Verification items for the finished model (mm, model axes). Face numbers are marked on the shaded views. A direction names the side the tool comes from. Coordinates: 2 decimals unless noted, no trailing zeros. Order: outer loops, then holes, each group sorted by start corner. A loop starts at its lowest first (then second) coordinate and runs counter-clockwise, first axis right, second up. Notation, with made-up numbers: (85.25, 48) -> (137.25, 48) arc R17 ccw to (137.25, 75) -> close; hole circle Ø9 at (-14, 66). An arc over 180 degrees is marked (long way). Answer as CSV lines item,"result".
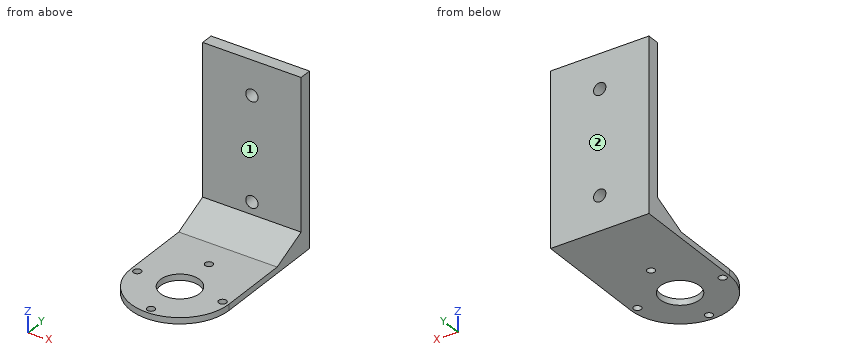
```python
from build123d import *

# Parameters (mm, degrees)
SKETCH1_R           = 10.16
SKETCH1_R_2         = 2
BOSS_EXTRUDE1_DEPTH = 3.175
SKETCH2_W           = 50.8
SKETCH2_H           = 88.9
SKETCH2_R           = 3.175
BOSS_EXTRUDE2_DEPTH = 6.35
BOSS_EXTRUDE3_DEPTH = 50.8


with BuildPart() as part:
    # Sketch1 → Boss-Extrude1 (new body)
    with BuildSketch(Plane.XY):
        with BuildLine():
            Line((-25.4, 0), (-25.4, 60.96))
            Line((-25.4, 60.96), (25.4, 60.96))
            Line((25.4, 60.96), (25.4, 0))
            ThreePointArc((25.4, 0), (0, -25.4), (-25.4, 0))
        make_face()
        Circle(SKETCH1_R, mode=Mode.SUBTRACT)
        with Locations((0, -22)):
            Circle(SKETCH1_R_2, mode=Mode.SUBTRACT)
        with Locations((-22, 0)):
            Circle(SKETCH1_R_2, mode=Mode.SUBTRACT)
        with Locations((0, 22)):
            Circle(SKETCH1_R_2, mode=Mode.SUBTRACT)
        with Locations((22, 0)):
            Circle(SKETCH1_R_2, mode=Mode.SUBTRACT)
    extrude(amount=BOSS_EXTRUDE1_DEPTH)

    # Sketch2 → Boss-Extrude2 (add)
    with BuildSketch(Plane(origin=(0, 60.96, 0), x_dir=(1, 0, 0), z_dir=(0, 1, 0))):
        with Locations((0, -44.45)):
            Rectangle(SKETCH2_W, SKETCH2_H)
        with Locations(Location((0, -17.78, 0), (0, 0, 270))):
            Circle(SKETCH2_R, mode=Mode.SUBTRACT)
        with Locations(Location((0, -71.12, 0), (0, 0, 270))):
            Circle(SKETCH2_R, mode=Mode.SUBTRACT)
    extrude(amount=-BOSS_EXTRUDE2_DEPTH)

    # Sketch3 → Boss-Extrude3 (add)
    with BuildSketch(Plane.ZY.offset(25.4)):
        Polygon((11.441642041, 54.61), (3.175, 36.439571989), (3.175, 54.61), align=None)
    extrude(amount=-BOSS_EXTRUDE3_DEPTH)


solid = part.part
```
Item 1: Section check C-C, the plane x = -6. Record the boundary of the cut face in (y, z) (3 decimals), plus the area to 3 significant figures.
Answer list:
outline,"(-24.681, 0) -> (-8.199, 0) -> (-8.199, 3.175) -> (-24.681, 3.175) -> close; (8.199, 0) -> (60.96, 0) -> (60.96, 88.9) -> (54.61, 88.9) -> (54.61, 11.442) -> (36.44, 3.175) -> (8.199, 3.175) -> close"
area,"839 mm2"
Item 2: Section check A-A, the plane y = 22. Record the boundary of the cut face in (x, z) (3 decimals), plus the area to 3 significant figures.
Answer list:
outline,"(-25.4, 0) -> (-2, 0) -> (-2, 3.175) -> (-25.4, 3.175) -> close; (2, 0) -> (25.4, 0) -> (25.4, 3.175) -> (2, 3.175) -> close"
area,"149 mm2"
Item 3: Depth check by flat-ended pin: pin 1 Ø6.5 at (x, y) = (-22, 0) entering from +Z (3 decimals); pin 2 Ø2.5 at (x, y) = (0, 22) entering from +Z; pin 3 Ø1 at (x, z) = (1, 26) entering from -Y. Enter the tip coordinate at first touch or a pass-through.
Answer list:
pin 1,"z = 3.175"
pin 2,"through"
pin 3,"y = 54.61"
Item 4: Thickness scan on line 1 (Y direction, x = 0, z = 1.6); line 2 (Z direction, x = 19, y = -9.5) (3 decimals); line 3 (Y direction, x = 18.5, z = 74.5). Record the ranges inside material, lowest first.
Answer list:
line 1,"-25.4 to -24, -20 to -10.16, 10.16 to 20, 24 to 60.96"
line 2,"0 to 3.175"
line 3,"54.61 to 60.96"
Item 5: Section check B-B, the plane x = 0. Record the boundary of the cut face in (y, z) (3 decimals).
Answer list:
outline,"(-25.4, 0) -> (-24, 0) -> (-24, 3.175) -> (-25.4, 3.175) -> close; (-20, 0) -> (-10.16, 0) -> (-10.16, 3.175) -> (-20, 3.175) -> close; (10.16, 0) -> (20, 0) -> (20, 3.175) -> (10.16, 3.175) -> close; (24, 0) -> (60.96, 0) -> (60.96, 14.605) -> (54.61, 14.605) -> (54.61, 11.442) -> (36.44, 3.175) -> (24, 3.175) -> close; (54.61, 20.955) -> (60.96, 20.955) -> (60.96, 67.945) -> (54.61, 67.945) -> close; (54.61, 74.295) -> (60.96, 74.295) -> (60.96, 88.9) -> (54.61, 88.9) -> close"
Item 6: Tool access check on the marked faces 1 and 2. Record the directions out of +Z, -Z, +X, -X, +Y, -Y that give a thin tool (end or side, any length) a straight path to the whole face; none if there is none.
Answer list:
face 1,"+Z, +X, -X, -Y"
face 2,"+Z, -Z, +X, -X, +Y"
Item 7: Section check D-D, the plane y = -22. Record the boundary of the cut face in (x, z) (3 decimals), plus the area to 3 significant figures.
Answer list:
outline,"(-12.695, 0) -> (-2, 0) -> (-2, 3.175) -> (-12.695, 3.175) -> close; (2, 0) -> (12.695, 0) -> (12.695, 3.175) -> (2, 3.175) -> close"
area,"67.9 mm2"
